Build history of the part. All positions in model axes, mm. Face numbers are marked on the shaded views. A direction names the side the tool comes from. Give positions to 0.01 mm unless a question says otherwise; leave off trailing zeros. Write each loop counter-clockwise with the first axis right and the second up, starting at its lowest first coordinate (ties: lowest second). Pieces come first, ordered by that corner, then holes.
from build123d import *

# Parameters (mm, degrees)
SKETCH_1_R          = 3.5
EXTRUDE_1_DEPTH     = 20
SKETCH_2_R          = 0.5
EXTRUDE_2_DEPTH     = 5
FILLET_1_R          = 0.3
SKETCH_3_R          = 0.25
CUT_EXTRUDE_1_DEPTH = 5
SKETCH_4_OUTSIDE_W  = 14.378
SKETCH_4_OUTSIDE_H  = 14.378
SKETCH_4_OUTSIDE_R  = 3
CUT_EXTRUDE_2_DEPTH = 0.3
SKETCH_5_R          = 0.5
CUT_EXTRUDE_3_DEPTH = 0.3


with BuildPart() as part:
    # 草图1 → 凸台-拉伸1 (new body)
    with BuildSketch(Plane(origin=(0, 0, 0), x_dir=(1, 0, 0), z_dir=(0, 1, 0))):
        Circle(SKETCH_1_R)
    extrude(amount=EXTRUDE_1_DEPTH)

    # 草图2 → 凸台-拉伸2 (add)
    with BuildSketch(Plane(origin=(0, 20, 0), x_dir=(1, 0, 0), z_dir=(0, 1, 0))):
        Circle(SKETCH_2_R)
    extrude(amount=EXTRUDE_2_DEPTH)

    # 圆角1
    fillet_1_edges = [part.edges().sort_by_distance(p)[0] for p in [
        (-3.5, 20, 0),
    ]]
    fillet(fillet_1_edges, radius=FILLET_1_R)

    # 草图3 → 切除-拉伸1 (cut)
    with BuildSketch(Plane(origin=(0, 20, 0), x_dir=(1, 0, 0), z_dir=(0, 1, 0))):
        with Locations((-1.414213562, 1.414213562)):
            Circle(SKETCH_3_R)
        with Locations((1.414213562, 1.414213562)):
            Circle(SKETCH_3_R)
        with Locations((1.414213562, -1.414213562)):
            Circle(SKETCH_3_R)
        with Locations((-1.414213562, -1.414213562)):
            Circle(SKETCH_3_R)
    extrude(amount=-CUT_EXTRUDE_1_DEPTH, mode=Mode.SUBTRACT)

    # 草图4 outside → 切除-拉伸2 (cut)
    with BuildSketch(Plane.XZ):
        Rectangle(SKETCH_4_OUTSIDE_W, SKETCH_4_OUTSIDE_H)
        Circle(SKETCH_4_OUTSIDE_R, mode=Mode.SUBTRACT)
    extrude(amount=-CUT_EXTRUDE_2_DEPTH, mode=Mode.SUBTRACT)

    # 草图5 → 切除-拉伸3 (cut)
    with BuildSketch(Plane.XZ):
        Circle(SKETCH_5_R)
    extrude(amount=-CUT_EXTRUDE_3_DEPTH, mode=Mode.SUBTRACT)


solid = part.part
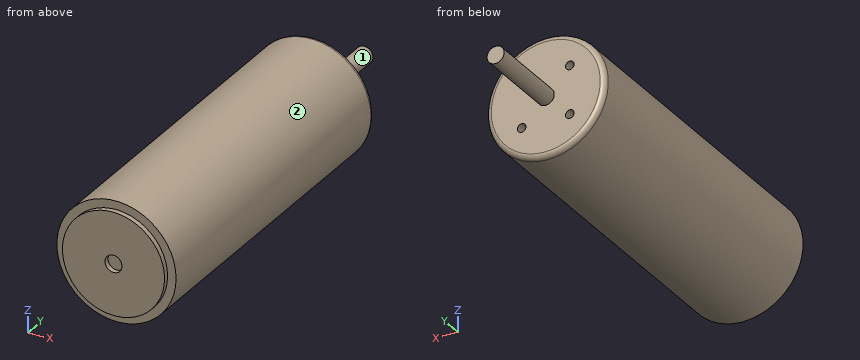
(1) Saw through at D-D, the plane y = 5.5. List the corners of the cut face in (x, z).
(2) Saw through at B-B, the plane x = 0. List the corners of the cut face in (y, z), plus the area to 3 significant figures.
(3) Saw through at A-A, the plane z = 0. List the corners of the cut face in (x, y), plus the area to 3 significant figures.
(4) Probe line 1 (Y direction, x = 0.5, z = -2); line 2 (Y direction, x = 1.75, z = -2.5); line 3 (X direction, y = 16, z = -2.75). List the from-to ranges inside material, lowest first.
(5) Drop flat-ended pins along their axis: pin 1 (1 mm diameter, centred on x = 2.5, y = 9.5, fed in from +Z); pin 2 (2 mm diameter, centred on x = 0.5, z = -2, fed in from +Y). Give the stop position or say it passes through.
(6) Saw through at C-C, the plane y = 17. List the corners of the cut face in (x, z).
(7) 3-axis set-ups, long thin cutter, end or side, ignore diameter. For the marked faces 1 and 2: which of +Z, -Z, +X, -X, +Y, -Y reach the whole face in a straight line?
Computed values:
1. outline: circle Ø7 at (0, 0)
2. outline: (0, -3) - (0.3, -3) - (0.3, -3.5) - (19.7, -3.5) arc R0.3 ccw to (20, -3.2) - (20, -0.5) - (25, -0.5) - (25, 0.5) - (20, 0.5) - (20, 3.2) arc R0.3 ccw to (19.7, 3.5) - (0.3, 3.5) - (0.3, 3) - (0, 3) - (0, 0.5) - (0.3, 0.5) - (0.3, -0.5) - (0, -0.5) - close
2. area: 144 mm2
3. outline: (-3.5, 0.3) - (-3, 0.3) - (-3, 0) - (-0.5, 0) - (-0.5, 0.3) - (0.5, 0.3) - (0.5, 0) - (3, 0) - (3, 0.3) - (3.5, 0.3) - (3.5, 19.7) arc R0.3 ccw to (3.2, 20) - (0.5, 20) - (0.5, 25) - (-0.5, 25) - (-0.5, 20) - (-3.2, 20) arc R0.3 ccw to (-3.5, 19.7) - close
3. area: 144 mm2
4. line 1: y = 0 to 20
4. line 2: y = 0.3 to 20
4. line 3: x = -2.17 to 2.17
5. pin 1: stops at z = 2.87
5. pin 2: stops at y = 20
6. outline: circle Ø7 at (0, 0); hole circle Ø0.5 at (-1.41, -1.41); hole circle Ø0.5 at (-1.41, 1.41); hole circle Ø0.5 at (1.41, -1.41); hole circle Ø0.5 at (1.41, 1.41)
7. face 1: +Y
7. face 2: +Y, -Y
